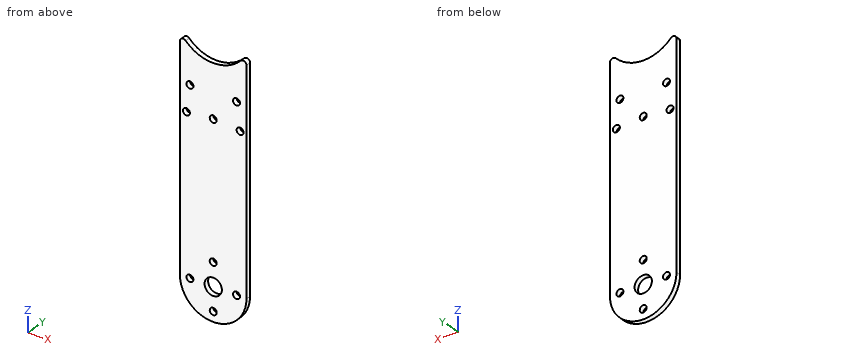
Autodesk Inventor part; units mm, degrees
ref_plane "YZ Plane" through (0, 0, 0) normal (1, 0, 0) x (0, 1, 0)
ref_plane "XZ Plane" through (0, 0, 0) normal (0, 1, 0) x (-1, 0, 0)
ref_plane "XY Plane" through (0, 0, 0) normal (0, 0, 1) x (1, 0, 0)
sketch "Sketch1" plane through (0, 0, 0) normal (0, 1, 0) x (-1, 0, 0)
  line L0 (10, -35) -> (-10, -35)
  line L1 (-10, -35) -> (-10, 44.4211)
  line L2 (10, 44.4211) -> (10, -35)
  arc A0 (-10, 44.4211) -> (10, 44.4211) centre (0, 50.1) ccw
  point P0 (0, 0)
  dimension "d2" = 35
  dimension "d3" = 10
  dimension "d36" = 23
  dimension "d37" = 85.1
  dimension "d39" = 79.4211
  dimension "d40" = 20
extrude "Plate1" add sketch "Sketch1" along normal blind 1.5
sketch "Sketch3" plane through (0, 1.5, 0) normal (0, 1, 0) x (1, 0, 0)
  circle A0 centre (0, 25) radius 10
  circle A1 centre (0, -25) radius 10
  line L0 (-10, 35) -> (10, 35)
  line L1 (10, -44) -> (-10, -44)
  line L2 (-10, 35) -> (10, 35)
  line L3 (10, 35) -> (10, 25)
  line L4 (10, 25) -> (-10, 25)
  line L5 (-10, 25) -> (-10, 35)
  line L6 (10, -35) -> (-10, -35)
  line L7 (-10, -35) -> (-10, -25)
  line L8 (-10, -25) -> (10, -25)
  line L9 (10, -25) -> (10, -44)
  point P0 (0, 0)
  point P1 (-10, -44.4211)
  point P2 (10, -25)
  point P3 (0, -35)
  point P4 (-10, -35)
  point P5 (0, 35)
  point P6 (10, 35)
  dimension "d12" = 20
  dimension "d13" = 20
  dimension "d14" = 10
  dimension "d15" = 10
  dimension "d16" = 25
  dimension "d17" = 25
  dimension "d18" = 10
extrude "Extrusion1" cut sketch "Sketch3" against normal blind 10 contours L5 L0 A0 | A0 L0 L3
sketch "Sketch4" plane through (0, 1.5, 0) normal (0, 1, 0) x (1, 0, 0)
  circle A0 centre (-7, 25) radius 0.8
  arc A1 (10, 25) -> (-10, 25) centre (0, 25) ccw
  circle A2 centre (0, 18) radius 0.8
  circle A3 centre (7, 25) radius 0.8
  circle A4 centre (0, 32) radius 0.8
  point P0 (0, 0)
  dimension "d21" = 0
  dimension "d22" = 7
  dimension "d23" = 1.6
  dimension "d26" = 360
hole "Hole2" at (0, 1.5, -32) at (7, 1.5, -25) at (0, 1.5, -18) at (-7, 1.5, -25) direction (0, -1, 0) diameter 2.1 depth 1.5
sketch "Sketch5" plane through (0, 1.5, 0) normal (0, 1, 0) x (1, 0, 0)
  arc A0 (10, 25) -> (-10, 25) centre (0, 25) ccw
  point P0 (0, 0)
hole "Hole3" at (0, 1.5, -25) direction (0, -1, 0) diameter 5.2 depth 1.5
fillet "Fillet1" radius 1 2 edges at (10, 0.75, 44.4211) (-10, 0.75, 44.4211)
sketch "Sketch7" plane through (0, 1.5, 0) normal (0, 1, 0) x (1, 0, 0)
  circle A0 centre (7, -29.98) radius 1.05
  circle A1 centre (8.07, -22) radius 1.05
  circle A2 centre (-7, -29.98) radius 1.05
  circle A3 centre (0, -22.68) radius 1.05
  circle A4 centre (-8.07, -22) radius 1.05
  point P0 (0, 0)
hole "Hole5" at (-8.07, 1.5, 22) at (0, 1.5, 22.68) at (8.07, 1.5, 22) at (7, 1.5, 29.98) at (-7, 1.5, 29.98) direction (0, -1, 0) diameter 2.1 end through all
equation "\"d33\" = Thickness"
equation "\"d46\" = Thickness"
equation "\"d61\" = Thickness"
equation "\"d4\" = Thickness"
equation "\"BendReliefWidth\" = Thickness"
equation "\"BendReliefDepth\" = 0.5 * Thickness"
equation "\"CornerReliefSize\" = 4 * Thickness"
equation "\"MinimumRemnant\" = 2 * Thickness"
equation "\"TransitionRadius\" = BendRadius"
equation "\"JacobiRadiusSize\" = BendRadius"
equation "\"GapSize\" = Thickness"
properties part number "axis_8_10_connector_frame" material "Aluminum 6061-AHC"
The listing builds one solid part. Answer for the finished solid, in the listing's coordinates (mm). Coordinates: 2 decimals unless noted, no trailing zeros. Loops run counter-clockwise (first coordinate to the right, second up) from the corner with the lowest first, then second, coordinate; pieces in that order, holes last. Notation, with made-up numbers: (25.5, 41) -> (39.5, 41) arc R23 ccw to (39.5, 63) -> close; hole circle Ø5 at (62.5, -16.75). An arc over 180 degrees is marked (long way). Write item = value, one per line. Start each with the question number.
1) Straight lines are drawn through the part: line 1 (X direction, y = 0.9, z = -25); line 2 (X direction, y = 1.35, z = -18); line 3 (X direction, y = 0.55, z = 22.68). For each, find the intervals that lie inside material, in ascending order. Write a range as from..to.
2) A cutting plane is placed at A-A (z = 29.98). Give the vertices of the cut face in (x, y), then the cut area to 3 significant figures.
3) A cutting plane is placed at C-C (x = 0). Give the vertices of the cut face in (y, z), then the cut area to 4 significant figures.
4) A cutting plane is placed at D-D (y = 0.55). Count the separate pieces of the cut face and the enclosed holes in it, then the cut area to 3 significant figures.
5) Given pin 1 Ø1.7 at (x, z) = (-7, -25) entering from +Y, flat-ended and moving along its own axis, determine where the tip first touches the part or whether it passes through.
6) A cutting plane is placed at B-B (z = -18). Give the vertices of the cut face in (x, y), then the cut area to 4 significant figures.
Responses:
q1.line_1 = -10..-8.05, -5.95..-2.6, 2.6..5.95, 8.05..10
q1.line_2 = -10..-1.05, 1.05..10
q1.line_3 = -10..-8.87, -7.27..-1.05, 1.05..7.27, 8.87..10
q2.outline = (-10, 0) -> (-8.05, 0) -> (-8.05, 1.5) -> (-10, 1.5) -> close; (-5.95, 0) -> (5.95, 0) -> (5.95, 1.5) -> (-5.95, 1.5) -> close; (8.05, 0) -> (10, 0) -> (10, 1.5) -> (8.05, 1.5) -> close
q2.area = 23.7 mm²
q3.outline = (0, -35) -> (1.5, -35) -> (1.5, -33.05) -> (0, -33.05) -> close; (0, -30.95) -> (1.5, -30.95) -> (1.5, -27.6) -> (0, -27.6) -> close; (0, -22.4) -> (1.5, -22.4) -> (1.5, -19.05) -> (0, -19.05) -> close; (0, -16.95) -> (1.5, -16.95) -> (1.5, 21.63) -> (0, 21.63) -> close; (0, 23.73) -> (1.5, 23.73) -> (1.5, 38.6) -> (0, 38.6) -> close
q3.area = 93.15 mm²
q4.separate_pieces = 1
q4.enclosed_holes = 10
q4.area = 1,410 mm²
q5.pin_1 = through
q6.outline = (-10, 0) -> (-1.05, 0) -> (-1.05, 1.5) -> (-10, 1.5) -> close; (1.05, 0) -> (10, 0) -> (10, 1.5) -> (1.05, 1.5) -> close
q6.area = 26.85 mm²
